Autodesk Inventor part; units mm, degrees
ref_plane "YZ Plane" through (0, 0, 0) normal (1, 0, 0) x (0, 1, 0)
ref_plane "XZ Plane" through (0, 0, 0) normal (0, 1, 0) x (-1, 0, 0)
ref_plane "XY Plane" through (0, 0, 0) normal (0, 0, 1) x (1, 0, 0)
sketch "Sketch1" plane through (0, 0, 0) normal (0, 0, 1) x (1, 0, 0)
  line L0 (-50.8, -44.45) -> (50.8, -44.45)
  line L1 (50.8, -44.45) -> (50.8, 44.45)
  line L2 (50.8, 44.45) -> (-50.8, 44.45)
  line L3 (-50.8, 44.45) -> (-50.8, -44.45)
  line L4 (-50.8, -44.45) -> (50.8, 44.45) construction
  line L5 (50.8, -44.45) -> (-50.8, 44.45) construction
  point P0 (0, 0)
  dimension "d0" = 101.6
  dimension "d1" = 88.9
extrude "Extrusion1" add sketch "Sketch1" along normal blind 50.8
sketch "Sketch2" plane through (0, 0, 50.8) normal (0, 0, 1) x (1, 0, 0)
  line L0 (50.8, 44.45) -> (-50.8, 44.45)
  line L1 (0, 44.45) -> (50.8, -16.0911) construction
  line L2 (50.8, -44.45) -> (50.8, 44.45)
  line L3 (0, 44.45) -> (79.0308, 44.45) construction
  line L4 (16.9102, 44.45) -> (50.8, 4.0618)
  line L5 (-16.9102, 44.45) -> (50.8, -36.2439)
  line L6 (-16.9102, 44.45) -> (16.9102, 44.45)
  line L7 (50.8, 4.0618) -> (50.8, -36.2439)
  point P0 (0, 0)
  dimension "d4" = 50
  dimension "d5" = 12.954
  dimension "d15" = 12.954
extrude "Extrusion2" cut sketch "Sketch2" against normal blind 25.908 contours L4 L2 L5 L0
sketch "Sketch3" plane through (0, 0, 50.8) normal (0, 0, 1) x (1, 0, 0)
  line L0 (50.8, -36.2439) -> (-16.9102, 44.45)
  line L1 (-50.8, 44.45) -> (-50.8, -44.45)
  line L2 (-50.8, 25.5652) -> (7.9497, -44.45)
  line L3 (-50.8, -44.45) -> (50.8, -44.45)
  line L4 (7.9497, -44.45) -> (-50.8, -44.45)
  line L5 (-50.8, -44.45) -> (-50.8, 25.5652)
  point P0 (0, 0)
  dimension "d16" = 38.1
extrude "Extrusion3" cut sketch "Sketch3" against normal through all
equation "\"d5\" = 0.5 * widthFor1inch"
equation "\"d15\" = 0.5 * widthFor1inch"
equation "\"d7\" = widthFor1inch"
equation "\"widthFor1inch\" = 25.908"
properties part number "jjig02"
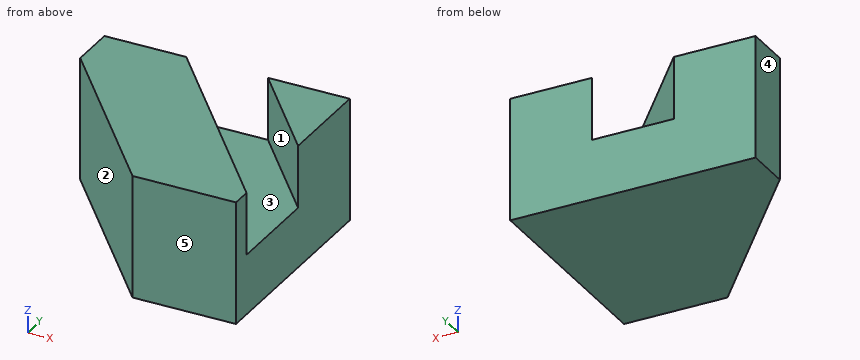
Geometry: final body of the model. Coordinates: model frame, mm. Face numbers are marked on the shaded views. A direction names the side the tool comes from. Give positions to 0.01 mm unless a question says otherwise; leave off trailing zeros. Loops run counter-clockwise (first coordinate to the right, second up) from the corner with the lowest first, then second, coordinate; pieces in that order, holes last. Notation, with made-up numbers: (-5, 35) -> (18, 35) arc R22 ccw to (18, 63) -> close; hole circle Ø8 at (70, 48.25). An arc over 180 degrees is marked (long way). Put each result on its own line as item: value.
1. Cut plane B-B (y = 39). Return the cut outline in (x, z).
Taken from the geometry:
outline: (-50.8, 0) -> (50.8, 0) -> (50.8, 50.8) -> (21.48, 50.8) -> (21.48, 24.89) -> (-12.34, 24.89) -> (-12.34, 50.8) -> (-50.8, 50.8) -> close
2. Pull-direction query (X, two-part tool) for the marked faces 3, 4 and 5; classes: released by +X, released by -X, zero draft, split by the parting line, or undercut.
Taken from the geometry:
face 3: undercut
face 4: released by -X
face 5: zero draft
3. Pin query (flat end, axial travel): P1, Ø1.5, axis at y = 15.5, z = 21.5, coming from the -X side; P2, Ø1, axis at x = -1.5, z = 44.5, coming from the -Y side; P3, Ø6, axis at x = 7, z = 9, coming from the -Y side. Return the tip coordinate at first contact, or that it passes through.
Taken from the geometry:
P1: stops at x = -42.98
P2: stops at y = -33.78
P3: stops at y = -44.45
4. Ray query, line 1 along X through (y, z) = (11, 37); line 2 along X through (y, z) = (27.5, 47.5); line 3 along Y through (x, z) = (25, 44). Return the intervals inside material, ascending. Write a range as [from, to].
Taken from the geometry:
line 1: x = [-38.58, 11.16], [44.98, 50.8]
line 2: x = [-50.8, -2.69], [31.13, 50.8]
line 3: y = [-44.45, -5.5], [34.81, 44.45]
5. Set-up query: the marked faces 1 and 2. Return all of +Z, -Z, +X, -X, +Y, -Y with unobstructed straight access to the full face (end or side cutting, diameter ignored); none if empty.
Taken from the geometry:
face 1: +Z
face 2: +Z, -Z, -X, -Y
6. Cut plane D-D (x = -15.5). Return the cut outline in (y, z), plus the area to 3 significant figures.
Taken from the geometry:
outline: (-16.5, 0) -> (44.45, 0) -> (44.45, 24.89) -> (42.77, 24.89) -> (42.77, 50.8) -> (-16.5, 50.8) -> close
area: 3,050 mm2
7. Cut plane A-A (z = 35.5). Return the cut outline in (x, y), plus the area to 3 significant figures.
Taken from the geometry:
outline: (-50.8, 25.57) -> (7.95, -44.45) -> (50.8, -44.45) -> (50.8, -36.24) -> (-16.91, 44.45) -> (-50.8, 44.45) -> close; (16.91, 44.45) -> (50.8, 4.06) -> (50.8, 44.45) -> close
area: 4,930 mm2
8. Cut plane C-C (z = 12). Return the cut outline in (x, y), plus the area to 3 significant figures.
Taken from the geometry:
outline: (-50.8, 25.57) -> (7.95, -44.45) -> (50.8, -44.45) -> (50.8, 44.45) -> (-50.8, 44.45) -> close
area: 6,980 mm2
